from build123d import *

# Parameters (mm, degrees)
MOUNTING_FLANGE_START                          = -4
SKETCH1_R                                      = 11
MOUNTING_FLANGE_DEPTH                          = 4
SKETCH2_R                                      = 2.75
D5P5_CENTRAL_POST_DEPTH                        = 31.01
CLOSED_FLOOR_BELOW_SHAFT_NOSE_START            = 31
SKETCH3_R                                      = 10
CLOSED_FLOOR_BELOW_SHAFT_NOSE_DEPTH            = 2
SHAFT_AND_CLIP_CLEARANCE_START                 = 33
SKETCH4_R                                      = 10
SKETCH4_R_2                                    = 5.7
SHAFT_AND_CLIP_CLEARANCE_DEPTH                 = 8.5
LOWER_686ZZ_SEAT_START                         = 41.5
SKETCH5_R                                      = 10
SKETCH5_R_2                                    = 6.5
LOWER_686ZZ_SEAT_DEPTH                         = 5
SKETCH6_R                                      = 1
BASE_THREE_M2_BLIND_THREAD_MAJOR_ENVELOP_DEPTH = 3.6
TOP_CAP_THREE_M2_BLIND_THREAD_MAJOR_ENVE_START = -4.3
SKETCH7_R                                      = 1
TOP_CAP_THREE_M2_BLIND_THREAD_MAJOR_ENVE_DEPTH = 4.3


with BuildPart() as part:
    # Sketch1 → Mounting_Flange (new body)
    with BuildSketch(Plane.XY.offset(MOUNTING_FLANGE_START)):
        Circle(SKETCH1_R)
    extrude(amount=MOUNTING_FLANGE_DEPTH)

    # Sketch2 → D5p5_Central_Post (add)
    with BuildSketch(Plane.XY):
        Circle(SKETCH2_R)
    extrude(amount=D5P5_CENTRAL_POST_DEPTH)

    # Sketch3 → Closed_Floor_Below_Shaft_Nose (add)
    with BuildSketch(Plane.XY.offset(CLOSED_FLOOR_BELOW_SHAFT_NOSE_START)):
        Circle(SKETCH3_R)
    extrude(amount=CLOSED_FLOOR_BELOW_SHAFT_NOSE_DEPTH)

    # Sketch4 → Shaft_And_Clip_Clearance (add)
    with BuildSketch(Plane.XY.offset(SHAFT_AND_CLIP_CLEARANCE_START)):
        Circle(SKETCH4_R)
        Circle(SKETCH4_R_2, mode=Mode.SUBTRACT)
    extrude(amount=SHAFT_AND_CLIP_CLEARANCE_DEPTH)

    # Sketch5 → Lower_686ZZ_Seat (add)
    with BuildSketch(Plane.XY.offset(LOWER_686ZZ_SEAT_START)):
        Circle(SKETCH5_R)
        Circle(SKETCH5_R_2, mode=Mode.SUBTRACT)
    extrude(amount=LOWER_686ZZ_SEAT_DEPTH)

    # Sketch6 → Base_Three_M2_Blind_Thread_Major_Envelopes (cut)
    with BuildSketch(Plane(origin=(0, 0, -4), x_dir=(-1, 0, 0), z_dir=(0, 0, -1))):
        with Locations((-7.188010851, 4.15)):
            Circle(SKETCH6_R)
        with Locations((7.188010851, 4.15)):
            Circle(SKETCH6_R)
        with Locations((0, -8.3)):
            Circle(SKETCH6_R)
    extrude(amount=-BASE_THREE_M2_BLIND_THREAD_MAJOR_ENVELOP_DEPTH, mode=Mode.SUBTRACT)

    # Sketch7 → Top_Cap_Three_M2_Blind_Thread_Major_Envelopes (cut)
    with BuildSketch(Plane.XY.offset(46.5).offset(TOP_CAP_THREE_M2_BLIND_THREAD_MAJOR_ENVE_START)):
        with Locations(Location((7.188010851, 4.15, 0), (0, 0, 180))):
            Circle(SKETCH7_R)
        with Locations(Location((-7.188010851, 4.15, 0), (0, 0, 180))):
            Circle(SKETCH7_R)
        with Locations(Location((0, -8.3, 0), (0, 0, 180))):
            Circle(SKETCH7_R)
    extrude(amount=TOP_CAP_THREE_M2_BLIND_THREAD_MAJOR_ENVE_DEPTH, mode=Mode.SUBTRACT)


solid = part.part
The listing builds one solid part. Answer for the finished solid, in the listing's coordinates (mm). A direction names the side the tool comes from. Give positions to 0.01 mm unless a question says otherwise; leave off trailing zeros. Write each loop counter-clockwise with the first axis right and the second up, starting at its lowest first coordinate (ties: lowest second). Pieces come first, ordered by that corner, then holes.
1) Section B-B (y = 0) is taken. Write down the section's boundary in (x, z).
2) Section C-C (y = -8.3) is taken. Write down the section's boundary in (x, z), and give its area (3 significant figures).
3) Section A-A (x = 0) is taken. Write down the section's boundary in (y, z).
4) Given P1, Ø12.5, axis at x = 1.5, y = 1, coming from the +Z side; P2, Ø4, axis at y = 1.5, z = 3, coming from the +X side; P3, Ø0.6, axis at x = -7.5, y = 4, coming from the +Z side; P4, Ø0.6, axis at x = 7, y = 4, coming from the -Z side, each flat-ended and moving along its own axis, determine where each tip first touches the part or whether it passes through.
5) Find the intervals of material crossed by L1, parallel to Z at x = 1.75, y = -4; L2, parallel to Z at x = -5.25, y = 7.5; L3, parallel to Y at x = 0, z = -2.3, in increasing order.
6) Section D-D (x = -4.5) is taken. Write down the section's boundary in (y, z).
7) For a pull along X with two mould halves and no side action, classify faces 1 (the face through (-0.596, -2.685, 15.283)), 2 (the face through (-4.5, -3.5, 37.2)), 3 (the face through (0, 0, -4)), 4 (the face through (0, 0, 33)) as pulls with the +X half, pulls with the -X half, needs draft (parallel to the pull), parting line crosses it, or undercut.
8) A tool of negligible diameter and unlimited length cuts with its end or side. For faces 5 (the face through (0, -7, 46.5)), 6 (the face through (-7, 4, 42.2)), 7 (the face through (2.3, -2.3, 0)), 8 (the face through (-6.394, 3.542, -2.225)), from which of +Z, -Z, +X, -X, +Y, -Y can it reach the whole face along a straight path? Write none if from no direction.
Response:
1. outline: (-11, -4) - (11, -4) - (11, 0) - (2.75, 0) - (2.75, 31) - (10, 31) - (10, 46.5) - (6.5, 46.5) - (6.5, 41.5) - (5.7, 41.5) - (5.7, 33) - (-5.7, 33) - (-5.7, 41.5) - (-6.5, 41.5) - (-6.5, 46.5) - (-10, 46.5) - (-10, 31) - (-2.75, 31) - (-2.75, 0) - (-11, 0) - close
2. outline: (-7.22, -4) - (-1, -4) - (-1, -0.4) - (1, -0.4) - (1, -4) - (7.22, -4) - (7.22, 0) - (-7.22, 0) - close; (-5.58, 31) - (5.58, 31) - (5.58, 46.5) - (1, 46.5) - (1, 42.2) - (-1, 42.2) - (-1, 46.5) - (-5.58, 46.5) - close
2. area: 215 mm2
3. outline: (-11, -4) - (-9.3, -4) - (-9.3, -0.4) - (-7.3, -0.4) - (-7.3, -4) - (11, -4) - (11, 0) - (2.75, 0) - (2.75, 31) - (10, 31) - (10, 46.5) - (6.5, 46.5) - (6.5, 41.5) - (5.7, 41.5) - (5.7, 33) - (-5.7, 33) - (-5.7, 41.5) - (-6.5, 41.5) - (-6.5, 46.5) - (-7.3, 46.5) - (-7.3, 42.2) - (-9.3, 42.2) - (-9.3, 46.5) - (-10, 46.5) - (-10, 31) - (-2.75, 31) - (-2.75, 0) - (-11, 0) - close
4. P1: stops at z = 46.5
4. P2: stops at x = 2.75
4. P3: stops at z = 42.2
4. P4: stops at z = -0.4
5. L1: z = -4 to 0, 31 to 33
5. L2: z = -4 to 0, 31 to 46.5
5. L3: y = -11 to -9.3, -7.3 to 11
6. outline: (-10.04, -4) - (10.04, -4) - (10.04, 0) - (-10.04, 0) - close; (-8.93, 31) - (8.93, 31) - (8.93, 46.5) - (4.69, 46.5) - (4.69, 41.5) - (3.5, 41.5) - (3.5, 33) - (-3.5, 33) - (-3.5, 41.5) - (-4.69, 41.5) - (-4.69, 46.5) - (-8.93, 46.5) - close
7. face 1: parting line crosses it
7. face 2: undercut
7. face 3: needs draft
7. face 4: undercut
8. face 5: +Z, +X, -X, +Y, -Y
8. face 6: +Z
8. face 7: none
8. face 8: -Z
